Read the model definition and answer for the solid it produces. Units are mm, in the model's axes. A direction names the side the tool comes from. Coordinates: 2 decimals unless noted, no trailing zeros. Loops run counter-clockwise (first coordinate to the right, second up) from the corner with the lowest first, then second, coordinate; pieces in that order, holes last. Notation, with made-up numbers: (87, -2.75) -> (123, -2.75) arc R20 cw to (123, 14.25) -> close; hole circle Ø8 at (45.25, 75.25). An arc over 180 degrees is marked (long way). Answer in a Markdown table with one row per item.
```python
from build123d import *

# Parameters (mm, degrees)
F0_R      = 86.75
F1_DEPTH  = 76.5
F2_R      = 110
F3_DEPTH  = 8.7
F4_R      = 110
F4_R_2    = 93.1
F4_R_3    = 89.1
F5_DEPTH  = 4
F6_R      = 93.1
F6_R_2    = 89.1
F7_DEPTH  = 4
F8_R      = 75
F9_DEPTH  = 73.1
F10_R     = 54.95
F11_DEPTH = 108.85
F12_R     = 44.95
F13_DEPTH = 49.55
F14_R     = 29.95
F15_DEPTH = 20
F16_R     = 25.95
F17_DEPTH = 39.3


with BuildPart() as f1:
    # F0 (on Top) → F1 (new body)
    with BuildSketch(Plane.XY):
        Circle(F0_R)
    extrude(amount=F1_DEPTH)

    # F2 (on face) → F3 (join)
    with BuildSketch(Plane.XY.offset(76.5)):
        Circle(F2_R)
    extrude(amount=-F3_DEPTH)

    # F4 (on face) → F5 (cut)
    with BuildSketch(Plane.XY.offset(76.5)):
        Circle(F4_R)
        Circle(F4_R_2, mode=Mode.SUBTRACT)
        Circle(F4_R_2)
        Circle(F4_R_3, mode=Mode.SUBTRACT)
    extrude(amount=-F5_DEPTH, mode=Mode.SUBTRACT)

    # F6 (on face) → F7 (cut)
    with BuildSketch(Plane.XY.offset(72.5)):
        Circle(F6_R)
        Circle(F6_R_2, mode=Mode.SUBTRACT)
    extrude(amount=-F7_DEPTH, mode=Mode.SUBTRACT)

    # F8 (on face) → F9 (cut)
    with BuildSketch(Plane.XY.offset(76.5)):
        Circle(F8_R)
    extrude(amount=-F9_DEPTH, mode=Mode.SUBTRACT)

    # F10 (on face) → F11 (join)
    with BuildSketch(Plane.XY.offset(3.4)):
        Circle(F10_R)
    extrude(amount=F11_DEPTH)

    # F12 (on face) → F13 (cut)
    with BuildSketch(Plane.XY.offset(112.25)):
        Circle(F12_R)
    extrude(amount=-F13_DEPTH, mode=Mode.SUBTRACT)

    # F14 (on face) → F15 (cut)
    with BuildSketch(Plane.XY.offset(62.7)):
        Circle(F14_R)
    extrude(amount=-F15_DEPTH, mode=Mode.SUBTRACT)

    # F16 (on face) → F17 (cut)
    with BuildSketch(Plane.XY.offset(42.7)):
        Circle(F16_R)
    extrude(amount=-F17_DEPTH, mode=Mode.SUBTRACT)


solid = f1.part
```
1. A tool of negligible diameter and unlimited length cuts with its end or side. For faces 4 (the flat face through (-1, 1, 0)), 5 (the cylindrical face through (-9.764, 74.362, 40.462)), 6 (the flat face through (81, 33, 67.8)), from which of +Z, -Z, +X, -X, +Y, -Y can it reach the whole face along a straight path? Write none if from no direction.
A:
| item | result |
|---|---|
| face 4 | -Z, +X, -X, +Y, -Y |
| face 5 | +Z |
| face 6 | -Z |
2. A cutting plane is placed at C-C on x = 64. Give the vertices of the cut face in (y, z).
A:
| item | result |
|---|---|
| outline | (-89.47, 67.8) -> (-58.56, 67.8) -> (-58.56, 0) -> (58.56, 0) -> (58.56, 67.8) -> (89.47, 67.8) -> (89.47, 72.5) -> (67.61, 72.5) -> (67.61, 68.5) -> (61.99, 68.5) -> (61.99, 76.5) -> (39.1, 76.5) -> (39.1, 3.4) -> (-39.1, 3.4) -> (-39.1, 76.5) -> (-61.99, 76.5) -> (-61.99, 68.5) -> (-67.61, 68.5) -> (-67.61, 72.5) -> (-89.47, 72.5) -> close |
3. A cutting plane is placed at A-A on z = 46.5. Give the vertices of the cut face in (x, y).
A:
| item | result |
|---|---|
| outline | circle Ø173.5 at (0, 0); circle Ø109.9 at (0, 0); hole circle Ø150 at (0, 0); hole circle Ø59.9 at (0, 0) |
4. Find the intervals of material crossed by probe 1 along X at (y, z) = (1, 40); probe 2 along Y at (x, z) = (0, 56); probe 3 along Y at (x, z) = (0, 42), in increasing order.
A:
| item | result |
|---|---|
| probe 1 | x = -86.74 to -74.99, -54.94 to -25.93, 25.93 to 54.94, 74.99 to 86.74 |
| probe 2 | y = -86.75 to -75, -54.95 to -29.95, 29.95 to 54.95, 75 to 86.75 |
| probe 3 | y = -86.75 to -75, -54.95 to -25.95, 25.95 to 54.95, 75 to 86.75 |
5. A cutting plane is placed at B-B on y = 70. Give the vertices of the cut face in (x, z), and give its area (3 significant figures).
A:
| item | result |
|---|---|
| outline | (-84.85, 67.8) -> (-51.24, 67.8) -> (-51.24, 0) -> (51.24, 0) -> (51.24, 67.8) -> (84.85, 67.8) -> (84.85, 72.5) -> (61.38, 72.5) -> (61.38, 68.5) -> (55.13, 68.5) -> (55.13, 76.5) -> (26.93, 76.5) -> (26.93, 3.4) -> (-26.93, 3.4) -> (-26.93, 76.5) -> (-55.13, 76.5) -> (-55.13, 68.5) -> (-61.38, 68.5) -> (-61.38, 72.5) -> (-84.85, 72.5) -> close |
| area | 4,200 mm2 |
6. Given pin 1 Ø1 at (x, y) = (34.5, 9.5) entering from +Z; pin 2 Ø6 at (y, z) = (-14.5, 73.5) entering from +X; pin 3 Ø6 at (x, y) = (-70.5, -78.5) entering from -Z, each flat-ended and moving along its own axis, determine where each tip first touches the part or whether it passes through.
A:
| item | result |
|---|---|
| pin 1 | stops at z = 62.7 |
| pin 2 | stops at x = 109.38 |
| pin 3 | stops at z = 67.8 |
7. The mould has two halves that part along Y. Classify faces 1 (the flat face through (29, -9, 62.7)), 2 (the flat face through (-47, -59, 76.5)), 3 (the cylindrical face through (-23.846, -107.384, 70.183)): pulls with the +Y half, pulls with the -Y half, needs draft (parallel to the pull), parting line crosses it, or undercut.
A:
| item | result |
|---|---|
| face 1 | undercut |
| face 2 | needs draft |
| face 3 | parting line crosses it |
